Build history of the part. All positions in model axes, mm. A direction names the side the tool comes from. Round coordinates to 2 decimals unless told otherwise and drop trailing zeros. Write each loop counter-clockwise with the first axis right and the second up, starting at its lowest first coordinate (ties: lowest second). Pieces come first, ordered by that corner, then holes.
Item 1: Mould opens along X. For faces 4 (the cylindrical face through (16.05, -0.69, -0.04)), 5 (the cylindrical face through (-5.85, -0.71, -0.03)), 6 (the flat face through (0, 0, 3)) say: +X half, -X half, draft (parallel to the pull), parting line (faces both ways), or undercut.
Item 2: Band-saw the part on C-C, the plane z = -1.5. Write the cut outline in (x, y), then the cut area to 3 significant figures.
Item 3: 3-axis set-ups, long thin cutter, end or side, ignore diameter. For faces 1 (the flat face through (-8.27, -0.69, -2.32)), 2 (the flat face through (1, -1.8, 1)), 3 (the flat face through (-1, -1, -1)): which of +Z, -Z, +X, -X, +Y, -Y reach the whole face in a straight line?
Item 4: Band-saw the part on D-D, the plane x = -1.5. Write the cut outline in (y, z).
Item 5: Band-saw the part on B-B, the plane x = -8.45. Write the cut outline in (y, z).
Item 6: Drop flat-ended pins along their axis: pin 1 Ø1.9 at (x, z) = (-8.45, 0) entering from +Y; pin 2 Ø1.1 at (x, z) = (4.45, 0) entering from -Y; pin 3 Ø1.4 at (x, z) = (-1, 0.5) entering from +Y; pin 4 Ø1 at (y, z) = (-1, -1) entering from -X. Give the stop position or say it passes through.
Item 7: Band-saw the part on A-A, the plane y = -0.4. Count the separate pieces of the cut face and the enclosed holes in it, then the cut area to 3 significant figures.
Item 8: Wall check: probe 1 along Y at (x, z) = (11, -1.5); probe 2 along Y at (x, z) = (-1.5, -1); probe 3 along Z at (x, y) = (-6.45, -0.45). Give the ranges that are in metal, low to high.
```python
from build123d import *

# Parameters (mm, degrees)
RESSALTO_EXTRUS_O1_DEPTH = 1.4
ESBO_O2_R                = 3.45
RESSALTO_EXTRUS_O2_DEPTH = 2.4
FURO4_D                  = 1.2
PADR_O_LINEAR1_COUNT     = 6
PADR_O_LINEAR1_PITCH     = 2
PADR_OCIRCULAR2_COUNT    = 2
PADR_OCIRCULAR2_COPY_1_D = 1.2
PADR_OCIRCULAR2_COPY_2_D = 1.2
PADR_OCIRCULAR2_COPY_3_D = 1.2
PADR_OCIRCULAR2_COPY_4_D = 1.2
PADR_OCIRCULAR2_COPY_5_D = 1.2
FURO1_D                  = 4.95
FURO1_DEPTH              = 2
FURO2_D                  = 4.6
FURO2_DEPTH              = 1
FURO3_D                  = 2.1
RESSALTO_EXTRUS_O3_DEPTH = 2


with BuildPart() as part:
    # Esboço1 → Ressalto-extrusão1 (new body)
    with BuildSketch(Plane(origin=(0, 0, 0), x_dir=(1, 0, 0), z_dir=(0, 1, 0))):
        with BuildLine():
            Line((-14.159121967, 1.99702088), (-2.209072203, 2.65))
            ThreePointArc((-2.209072203, 2.65), (3.45, 0), (-2.209072203, -2.65))
            Line((-2.209072203, -2.65), (-14.159121967, -1.99702088))
            ThreePointArc((-14.159121967, -1.99702088), (-16.05, 0), (-14.159121967, 1.99702088))
        make_face()
    ressalto_extrus_o1 = extrude(amount=-RESSALTO_EXTRUS_O1_DEPTH)

    # Esboço2 → Ressalto-extrusão2 (add)
    with BuildSketch(Plane.XZ.offset(1.4)):
        Circle(ESBO_O2_R)
    extrude(amount=RESSALTO_EXTRUS_O2_DEPTH)

    # Furo4 (through all)
    with Locations(Plane(origin=(0, 0, 0), x_dir=(1, 0, 0), z_dir=(0, 1, 0))):
        with Locations((-14.45, 0)):
            furo4 = Hole(FURO4_D / 2)

    # Padrão linear1: Furo4 ×6
    with Locations(*[(i * PADR_O_LINEAR1_PITCH, 0, 0) for i in range(1, PADR_O_LINEAR1_COUNT)]):
        add(furo4, mode=Mode.SUBTRACT)

    # PadrãoCircular2: Ressalto-extrusão1, Furo4 ×2 about axis
    padr_ocircular2_axis = Axis((0, 0, 0), (0, 1, 0))
    for i in range(1, PADR_OCIRCULAR2_COUNT):
        add(ressalto_extrus_o1.rotate(padr_ocircular2_axis, i * 360 / PADR_OCIRCULAR2_COUNT))
        add(furo4.rotate(padr_ocircular2_axis, i * 360 / PADR_OCIRCULAR2_COUNT), mode=Mode.SUBTRACT)

    # PadrãoCircular2 copy 1 (through all)
    with Locations(Plane(origin=(-2, 0, 0), x_dir=(-1, 0, 0), z_dir=(0, 1, 0))):
        with Locations((-14.45, 0)):
            Hole(PADR_OCIRCULAR2_COPY_1_D / 2)

    # PadrãoCircular2 copy 2 (through all)
    with Locations(Plane(origin=(-4, 0, 0), x_dir=(-1, 0, 0), z_dir=(0, 1, 0))):
        with Locations((-14.45, 0)):
            Hole(PADR_OCIRCULAR2_COPY_2_D / 2)

    # PadrãoCircular2 copy 3 (through all)
    with Locations(Plane(origin=(-6, 0, 0), x_dir=(-1, 0, 0), z_dir=(0, 1, 0))):
        with Locations((-14.45, 0)):
            Hole(PADR_OCIRCULAR2_COPY_3_D / 2)

    # PadrãoCircular2 copy 4 (through all)
    with Locations(Plane(origin=(-8, 0, 0), x_dir=(-1, 0, 0), z_dir=(0, 1, 0))):
        with Locations((-14.45, 0)):
            Hole(PADR_OCIRCULAR2_COPY_4_D / 2)

    # PadrãoCircular2 copy 5 (through all)
    with Locations(Plane(origin=(-10, 0, 0), x_dir=(-1, 0, 0), z_dir=(0, 1, 0))):
        with Locations((-14.45, 0)):
            Hole(PADR_OCIRCULAR2_COPY_5_D / 2)

    # Furo1
    with Locations(Plane(origin=(0, -3.8, 0), x_dir=(-1, 0, 0), z_dir=(0, -1, 0))):
        with Locations((0, 0)):
            Hole(FURO1_D / 2, depth=FURO1_DEPTH)

    # Furo2
    with Locations(Plane(origin=(0, 0, 0), x_dir=(1, 0, 0), z_dir=(0, 1, 0))):
        with Locations((0, 0)):
            Hole(FURO2_D / 2, depth=FURO2_DEPTH)

    # Furo3 (through all)
    with Locations(Plane(origin=(0, 0, 0), x_dir=(1, 0, 0), z_dir=(0, 1, 0))):
        with Locations((0, 0)):
            Hole(FURO3_D / 2)

    # Esboço11 → Ressalto-extrusão3 (add)
    with BuildSketch(Plane.XZ.offset(3.8)):
        with BuildLine():
            Line((-0.098056786, 2.473056786), (0, 2.375))
            Line((0, 2.375), (0.098056786, 2.473056786))
            ThreePointArc((0.098056786, 2.473056786), (0, 2.475), (-0.098056786, 2.473056786))
        make_face()
    extrude(amount=-RESSALTO_EXTRUS_O3_DEPTH)


solid = part.part
```
Results:
1. face 4: +X half
1. face 5: undercut
1. face 6: draft
2. outline: (-15.37, -1.4) - (-3.11, -1.4) - (-3.11, -3.8) - (-1.97, -3.8) - (-1.97, -1.8) - (1.97, -1.8) - (1.97, -3.8) - (3.11, -3.8) - (3.11, -1.4) - (15.37, -1.4) - (15.37, 0) - (1.74, 0) - (1.74, -1) - (-1.74, -1) - (-1.74, 0) - (-15.37, 0) - close
2. area: 46.6 mm2
3. face 1: -Z, -X, +Y, -Y
3. face 2: -Y
3. face 3: +Y
4. outline: (-3.8, -3.11) - (0, -3.11) - (0, -1.74) - (-1, -1.74) - (-1, 1.74) - (0, 1.74) - (0, 3.11) - (-3.8, 3.11) - (-3.8, 1.97) - (-1.8, 1.97) - (-1.8, -1.97) - (-3.8, -1.97) - close
5. outline: (-1.4, -2.31) - (0, -2.31) - (0, -0.6) - (-1.4, -0.6) - close; (-1.4, 0.6) - (0, 0.6) - (0, 2.31) - (-1.4, 2.31) - close
6. pin 1: stops at y = 0
6. pin 2: passes through
6. pin 3: stops at y = -1
6. pin 4: stops at x = -15.99
7. separate pieces: 1
7. enclosed holes: 13
7. area: 121 mm2
8. probe 1: y = -1.4 to 0
8. probe 2: y = -1.8 to -1
8. probe 3: z = -2.42 to -0.6, 0.6 to 2.42
